from build123d import *

# Parameters (mm, degrees)
SKETCH1_W           = 74
SKETCH1_H           = 14
SKETCH1_R           = 2.3
SKETCH1_W_2         = 53
SKETCH1_H_2         = 20
BOSS_EXTRUDE1_DEPTH = 5.2
CUT_EXTRUDE1_DEPTH  = 1
BOSS_EXTRUDE2_START = 7.2
BOSS_EXTRUDE2_DEPTH = 7.2
SKETCH5_R           = 1.55
CUT_EXTRUDE2_DEPTH  = 78.278781046
SKETCH6_W           = 34
SKETCH6_H           = 0.2
CUT_EXTRUDE3_DEPTH  = 78.651529283


with BuildPart() as part:
    # Sketch1 → Boss-Extrude1 (new body)
    # profile 1 of 2: a face of its own
    with BuildSketch(Plane(origin=(0, 0, 0), x_dir=(1, 0, 0), z_dir=(0, 1, 0))):
        with Locations((37, 7)):
            Rectangle(SKETCH1_W, SKETCH1_H)
        with Locations(Location((5, 7, 0), (0, 0, 270))):
            Circle(SKETCH1_R, mode=Mode.SUBTRACT)
        with Locations(Location((69, 7, 0), (0, 0, 270))):
            Circle(SKETCH1_R, mode=Mode.SUBTRACT)
    # profile 2 of 2: a face of its own
    with BuildSketch(Plane(origin=(0, 0, 0), x_dir=(1, 0, 0), z_dir=(0, 1, 0))):
        with Locations((37, -10)):
            Rectangle(SKETCH1_W_2, SKETCH1_H_2)
    extrude(amount=BOSS_EXTRUDE1_DEPTH)

    # Sketch2 → Cut-Extrude1 (cut)
    with BuildSketch(Plane(origin=(0, 5.2, 0), x_dir=(1, 0, 0), z_dir=(0, 1, 0))):
        with BuildLine():
            ThreePointArc((37, -5.85), (34.772613639, -6.772613639), (33.85, -9))
            Line((33.85, -9), (33.85, -20))
            Line((33.85, -20), (40.15, -20))
            Line((40.15, -20), (40.15, -9))
            ThreePointArc((40.15, -9), (39.227386361, -6.772613639), (37, -5.85))
        make_face()
    extrude(amount=-CUT_EXTRUDE1_DEPTH, mode=Mode.SUBTRACT)

    # Sketch3 → Boss-Extrude2 (add)
    with BuildSketch(Plane(origin=(0, 5.2, 0), x_dir=(1, 0, 0), z_dir=(0, 1, 0)).offset(BOSS_EXTRUDE2_START)):
        with BuildLine():
            Line((33.85, -9), (33.85, -16))
            Line((33.85, -16), (17, -16))
            Line((17, -16), (17, -4.5))
            Line((17, -4.5), (57, -4.5))
            Line((57, -4.5), (57, -16))
            Line((57, -16), (40.15, -16))
            Line((40.15, -16), (40.15, -9))
            ThreePointArc((40.15, -9), (37, -5.85), (33.85, -9))
        make_face()
    extrude(amount=-BOSS_EXTRUDE2_DEPTH)

    # Sketch5 → Cut-Extrude2 (cut, through all)
    with BuildSketch(Plane(origin=(0, 0, 4.5), x_dir=(-1, 0, 0), z_dir=(0, 0, -1))):
        with Locations((-52.45, 8.8)):
            Circle(SKETCH5_R)
        with Locations((-21.55, 8.8)):
            Circle(SKETCH5_R)
    extrude(amount=-CUT_EXTRUDE2_DEPTH, mode=Mode.SUBTRACT)

    # Sketch6 → Cut-Extrude3 (cut, through all)
    with BuildSketch(Plane.ZY):
        with Locations((3, 0.1)):
            Rectangle(SKETCH6_W, SKETCH6_H)
    extrude(amount=-CUT_EXTRUDE3_DEPTH, mode=Mode.SUBTRACT)


solid = part.part
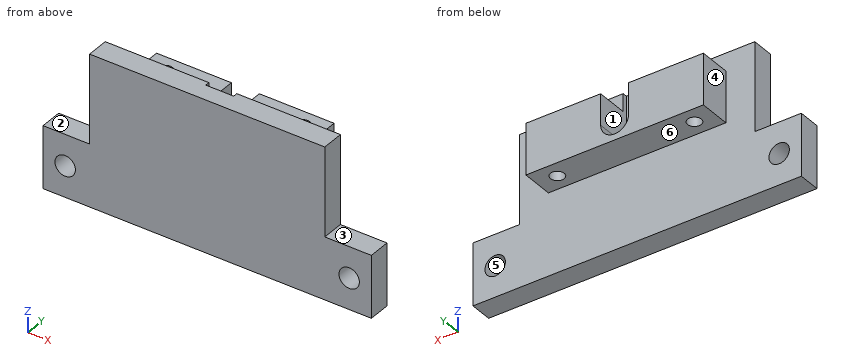
For this review, take the finished solid that the model builds, in its own axes (mm). Face numbers are marked on the shaded views. A direction names the side the tool comes from. Round coordinates to 2 decimals unless told otherwise and drop trailing zeros. Loops run counter-clockwise (first coordinate to the right, second up) from the corner with the lowest first, then second, coordinate; pieces in that order, holes last. Notation, with made-up numbers: (37.5, 16) - (74.5, 16) arc R18 ccw to (74.5, 51) - close; hole circle Ø11 at (-24.75, -21). An arc over 180 degrees is marked (long way). One line per question, with ' | ' between items.
Q1. The part is to be moulded in two halves that separate along Z. For the marked faces 4, 5 and 6, say which applies: released by +Z, released by -Z, zero draft, split by the parting line, or undercut.
Taken from the geometry:
face 4: zero draft | face 5: undercut | face 6: released by -Z
Q2. For line 1 along X through (y, z) = (1.9, -7); line 2 along Y through (x, z) = (26, 1.5); line 3 along X through (y, z) = (2.5, 1), list the stretches that pass through material, from the lowest coordinate up. Write a range as [from, to].
Taken from the geometry:
line 1: x = [0, 2.7], [7.3, 66.7], [71.3, 74] | line 2: y = [0.2, 5.2] | line 3: x = [10.5, 63.5]
Q3. Take a section at A-A (z = -7). Give the boundary of the cut face in (x, y).
Taken from the geometry:
outline: (0, 0.2) - (2.7, 0.2) - (2.7, 5.2) - (0, 5.2) - close; (7.3, 0.2) - (66.7, 0.2) - (66.7, 5.2) - (7.3, 5.2) - close; (71.3, 0.2) - (74, 0.2) - (74, 5.2) - (71.3, 5.2) - close
Q4. Take a section at C-C (y = 3). Give the boundary of the cut face in (x, z).
Taken from the geometry:
outline: (0, -14) - (74, -14) - (74, 0) - (63.5, 0) - (63.5, 20) - (10.5, 20) - (10.5, 0) - (0, 0) - close; hole circle Ø4.6 at (5, -7); hole circle Ø4.6 at (69, -7)
Q5. Take a section at D-D (x = 44). Give the boundary of the cut face in (y, z), and give its area (3 significant figures).
Taken from the geometry:
outline: (0.2, -14) - (5.2, -14) - (5.2, 4.5) - (12.4, 4.5) - (12.4, 16) - (5.2, 16) - (5.2, 20) - (0.2, 20) - close | area: 253 mm²
Q6. Take a section at B-B (x = 52.45). Give the boundary of the cut face in (y, z).
Taken from the geometry:
outline: (0.2, -14) - (5.2, -14) - (5.2, 4.5) - (7.25, 4.5) - (7.25, 16) - (5.2, 16) - (5.2, 20) - (0.2, 20) - close; (10.35, 4.5) - (12.4, 4.5) - (12.4, 16) - (10.35, 16) - close
Q7. Tool access review of the marked faces 1, 2 and 3: name each direction out of +Z, -Z, +X, -X, +Y, -Y from which nothing blocks a thin tool from reaching the whole face with its end or side.
Taken from the geometry:
face 1: +Z, +Y | face 2: +Z, -X, +Y, -Y | face 3: +Z, +X, +Y, -Y
Q8. For pin 1 (4 mm diameter, centred on x = 66.5, y = 2, fed in from +Z); pin 2 (6 mm diameter, centred on x = 46.5, y = 9.5, fed in from +Z); pin 3 (3 mm diameter, centred on x = 12, z = 10, fed in from +Y); pin 4 (3 mm diameter, centred on x = 69, z = -7, fed in from -Y), all flat-tipped, find the tip position at first contact; note any pin that passes through.
Taken from the geometry:
pin 1: stops at z = 0 | pin 2: stops at z = 16 | pin 3: stops at y = 5.2 | pin 4: passes through
